Could you check a few things on this model? Use its own coordinates, in mm. A direction names the side the tool comes from. Round coordinates to 2 decimals unless told otherwise and drop trailing zeros. Write each loop counter-clockwise with the first axis right and the second up, starting at its lowest first coordinate (ties: lowest second). Pieces come first, ordered by that corner, then holes. Notation, with made-up numbers: (79, -16.75) -> (121, -16.75) arc R29 ccw to (121, 4.25) -> close; hole circle Ø8 at (57, -12.75). An arc over 180 degrees is marked (long way). Return JSON: item names as keys, results as strings.
from build123d import *

# Parameters (mm, degrees)
F0_R     = 19.05
F1_DEPTH = 304.8
F3_SIZE  = 12.7
F4_DEPTH = 25.4
F5_T     = 2.54
F6_W     = 31.75
F6_H     = 19.05
F7_DEPTH = 5.08
F8_R     = 9.7478523701
F9_DEPTH = 25.4


with BuildPart() as f1:
    # F0 (on Front) → F1 (new body)
    with BuildSketch(Plane.XZ):
        Circle(F0_R)
    extrude(amount=F1_DEPTH)

    # F3
    f3_edges = [f1.edges().sort_by_distance(p)[0] for p in [
        (-19.05, 0, 0),
    ]]
    chamfer(f3_edges, length=F3_SIZE)

    # F4 (add): a face of the model
    f4_faces = [f1.faces().sort_by_distance(p)[0] for p in [
        (0, 0, 0),
    ]]
    extrude(f4_faces, amount=F4_DEPTH)

    # F5
    f5_openings = [f1.faces().sort_by_distance(p)[0] for p in [
        (0, -304.8, 0),
    ]]
    offset(amount=F5_T, openings=f5_openings, kind=Kind.INTERSECTION)


with BuildPart() as f7:
    # F6 (on face) → F7 (new body)
    with BuildSketch(Plane.XZ.offset(304.8)):
        Rectangle(F6_W, F6_H)
    extrude(amount=F7_DEPTH)


with BuildPart() as f9:
    # F8 (on face) → F9 (new body)
    with BuildSketch(Plane.XZ.offset(309.88)):
        Circle(F8_R)
    extrude(amount=-F9_DEPTH)


solid = f1.part
1) If I drill on probe 1 along Z at (x, y) = (0, 17); probe 2 along Z at (x, y) = (-1, -84), over which ranges is the centre line in solid material (lowest first)? Write a range as [from, to].
Return value:
{"probe 1": "[-8.89, -6.35], [6.35, 8.89]", "probe 2": "[-21.57, -19.02], [19.02, 21.57]"}
2) I want a section at C-C, the plane x = 0. Please give me the cut outline in (y, z), and give its area (3 significant figures).
Return value:
{"outline": "(-304.8, -21.59) -> (-11.65, -21.59) -> (1.05, -8.89) -> (27.94, -8.89) -> (27.94, 8.89) -> (1.05, 8.89) -> (-11.65, 21.59) -> (-304.8, 21.59) -> (-304.8, 19.05) -> (-12.7, 19.05) -> (0, 6.35) -> (25.4, 6.35) -> (25.4, -6.35) -> (0, -6.35) -> (-12.7, -19.05) -> (-304.8, -19.05) -> close", "area": "1,750 mm²"}
3) Thinking about a two-plate mould opening in X: for faces 4 (the face through (9.068, 0.435, 2.856)), 5 (the face through (0, 25.4, 0)), 6 (the face through (0, 27.94, 0)), which applies, pulls with the +X half, pulls with the -X half, needs draft (parallel to the pull), parting line crosses it, or undercut?
Return value:
{"face 4": "parting line crosses it", "face 5": "undercut", "face 6": "needs draft"}
4) I want a section at A-A, the plane z = 0. Please give me the cut outline in (x, y).
Return value:
{"outline": "(-21.59, -304.8) -> (-19.05, -304.8) -> (-19.05, -12.7) -> (-6.35, 0) -> (-6.35, 25.4) -> (6.35, 25.4) -> (6.35, 0) -> (19.05, -12.7) -> (19.05, -304.8) -> (21.59, -304.8) -> (21.59, -11.65) -> (8.89, 1.05) -> (8.89, 27.94) -> (-8.89, 27.94) -> (-8.89, 1.05) -> (-21.59, -11.65) -> close"}
5) For faces 1 (the face through (6.057, 12.522, 1.907)), 2 (the face through (-1.93, 14.31, -8.68)), 3 (the face through (-15.913, -156.172, 14.592)), which set-ups out of +Z, -Z, +X, -X, +Y, -Y let a thin tool reach every point of the face, with its end or its side?
Return value:
{"face 1": "-Y", "face 2": "+Y", "face 3": "+Y, -Y"}
6) Will these pins go through, and if not, where does the flat tip stop? pin 1 Ø2 at (y, z) = (-163, 5.5) entering from -X; pin 2 Ø10 at (y, z) = (-211, 6.5) entering from +X; pin 3 Ø3 at (x, z) = (-13, -11.5) entering from +Y.
Return value:
{"pin 1": "x = -21.12", "pin 2": "x = 21.54", "pin 3": "y = -5.91"}
7) I want a section at B-B, the plane y = -86. Please give me the cut outline in (x, z), and give its area (3 significant figures).
Return value:
{"outline": "circle Ø43.18 at (0, 0); hole circle Ø38.1 at (0, 0)", "area": "324 mm²"}
